Source: CAD feature listing. Evaluate the final solid. Frame: model axes, mm. Face numbers are marked on the shaded views. Give positions to 0.01 mm unless a question says otherwise; leave off trailing zeros. Write item = value, one per line.
Autodesk Inventor part; units mm, degrees
ref_plane "Work Plane2" through (-6.6501, -24.5518, 27.7072) normal (0, -0.0032, 1) x (1, 0, 0)
ref_plane "Work Plane3" through (-6.6501, -24.5518, 27.7072) normal (0, -0.0032, 1) x (1, 0, 0)
ref_plane "YZ Plane" through (0, 0, 0) normal (1, 0, 0) x (0, 1, 0)
ref_plane "Work Plane1" through (0, 0, 0) normal (0, 0, 1) x (1, 0, 0)
sketch "Sketch1" plane through (0, 0, 0) normal (0, 0, 1) x (1, 0, 0)
  spline S0 degree 3 poles (0.756, 49.6264) (0.8045, 49.3961) (1.4299, 46.4448) (3.02, 38.5419) (3.7417, 34.8308) (6.1255, 22.1808) (7.7131, 13.0519) (12.377, -15.9979) (15.3565, -38.2776) (18.0982, -72.579) (18.7462, -87.3982) (17.8341, -109.2065) (16.9191, -121.3453) (13.1344, -135.1445) (11.7229, -139.4741) (8.6906, -144.8131) (7.5566, -146.4347) (5.361, -148.5489) (4.4031, -149.2519) (2.172, -150.2514) (1.1579, -150.3736) (0.378, -150.3736) knots -21.570573 -21.570573 -21.570573 -21.570573 -20.133907 -20.133907 -18.864962 -18.864962 -15.766925 -15.766925 -8.908038 -8.908038 -4.28709 -4.28709 -1.655649 -1.655649 -0.852769 -0.852769 -0.490947 -0.490947 -0.258162 -0.258162 0 0 0 0
  line L0 (13.2039, -25.771) -> (-6.8, -25.771)
  line L1 (-6.8, 0) -> (9.8005, 0)
  line L2 (5.2, -2.2181) -> (5.2, 1.2819)
  line L3 (6.2, 0) -> (6.2, -25.771)
  line L4 (6.2, -0.25) -> (9.8396, -0.25)
  line L5 (6.2, -25.521) -> (13.4551, -25.521)
  circle A0 centre (8.0198, -0.25) radius 1
  circle A1 centre (8.0783, -25.521) radius 1
  circle A2 centre (8.0198, -0.25) radius 1
  circle A3 centre (8.0783, -25.521) radius 1
  point P0 (0, 0)
  point P1 (9.0783, -25.521)
  point P2 (9.0198, -0.25)
  point P3 (7.0198, -0.25)
  point P4 (7.0783, -25.521)
  dimension "d0" = 1
  dimension "d1" = 0.25
  dimension "d2" = 0.25
  dimension "d3" = 2
  dimension "d4" = 2
ref_plane "Work Plane2" through (-6.6501, -24.5518, 27.7072) normal (0, -0.0032, 1) x (1, 0, 0)
ref_plane "Work Plane3" through (-6.6501, -24.5518, 27.7072) normal (0, -0.0032, 1) x (1, 0, 0)
extrude "Extrusion1" add sketch "Sketch1" along normal up to surface contours S0 L5 A1 L3 L4 A0 | A0 L4 | L5 A1 surface through (-6.6501, -24.5518, 27.7072) normal (0, -0.0032, 1)
ref_plane "Work Plane4" through (0, 0, 80) normal (0, 0, 1) x (1, 0, 0)
sketch "Sketch3" plane through (6.2, -0.25, 0) normal (0, 1, 0) x (1, 0, 0)
  circle A0 centre (1.8198, -5) radius 1
  circle A1 centre (1.8198, -17.7838) radius 1
  line L0 (0, -27.7838) -> (3.6396, -27.7838)
  line L1 (3.6396, 0) -> (0, 0)
  point P0 (-6.2, 0)
  point P1 (1.8198, -27.7838)
  point P2 (1.8198, 0)
  dimension "d10" = 2
  dimension "d11" = 2
  dimension "d13" = 10
  dimension "d14" = 5
extrude "Extrusion3" add sketch "Sketch3" along normal blind 1
fillet "Fillet1" radius 1 2 edges at (7.0198, 0.75, 5) (7.0198, 0.75, 17.7838)
ref_plane "Work Plane5" through (6.2, -12.8855, 0) normal (0, 1, 0) x (1, 0, 0)
mirror "Mirror2" about plane through (6.2, -12.8855, 0) normal (0, 1, 0) of "Extrusion3"
fillet "Fillet2" radius 1 2 edges at (7.0198, -26.521, 17.7838) (7.0198, -26.521, 5)
ref_plane "Work Plane6" through (0, 0, 792.194) normal (0, 0, 1) x (1, 0, 0)
properties part number "servo cap"
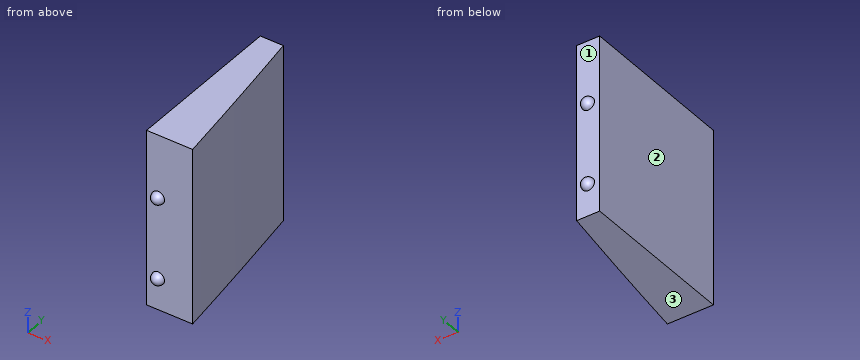
1) Material intervals for L1, parallel to Z at x = 9.75, y = -1.5; L2, parallel to Y at x = 9.75, z = 26.5; L3, parallel to Z at x = 7.75, y = -24.25, sorted ascending.
Computed:
L1 = 0 to 27.78
L2 = -25.52 to -0.25
L3 = 0 to 27.71
2) Contact query for flat-ended pins moving along their axis: pin 1 (1 mm diameter, centred on x = 9.5, z = 13.5, fed in from -Y); pin 2 (3 mm diameter, centred on x = 9, z = 13, fed in from +Y); pin 3 (3 mm diameter, centred on x = 7, y = -15, fed in from +Z). Output: stop coordinate, or through.
Computed:
pin_1 = -25.52
pin_2 = -0.25
pin_3 = 27.74
3) Draft query along Z for the marked faces 1, 2 and 3. Return one class per face: pulls with the +Z half, pulls with the -Z half, needs draft (parallel to the pull), parting line crosses it, or undercut.
Computed:
face_1 = undercut
face_2 = needs draft
face_3 = pulls with the -Z half
